```python
from build123d import *

# Parameters (mm, degrees)
F0_W     = 140
F0_H     = 15
F0_R     = 1.75
F1_DEPTH = 2.5
F3_DEPTH = 25
F4_W     = 18
F4_H     = 2.6
F4_W_2   = 12
F4_H_2   = 6
F4_W_3   = 10
F4_H_3   = 5
F5_DEPTH = 25
F6_D     = 3.4
F7_D     = 5.5
F8_R     = 5


with BuildPart() as f1:
    # F0 (on Top) → F1 (new body)
    with BuildSketch(Plane.XY):
        Rectangle(F0_W, F0_H)
        with Locations((-62, 0)):
            Circle(F0_R, mode=Mode.SUBTRACT)
        with Locations((62, 0)):
            Circle(F0_R, mode=Mode.SUBTRACT)
    extrude(amount=F1_DEPTH)

    # F2 (on face) → F3 (join)
    with BuildSketch(Plane.XY.offset(2.5)):
        Polygon((56.1840869486, 1.1), (-55.1196709275, 1.1), (-55.1196709275, -1.1), (56.1840869486, -1.1), (56.1840869486, 0), align=None)
    extrude(amount=F3_DEPTH)

    # F4 (on face) → F5 (cut)
    with BuildSketch(Plane(origin=(0, 1.1, 0), x_dir=(-1, 0, 0), z_dir=(0, 1, 0))):
        with Locations((42.6196709275, 16.3)):
            Rectangle(F4_W, F4_H)
        with Locations((42.6196709275, 13.7)):
            Rectangle(F4_W, F4_H)
        with Locations((15.6196709275, 18)):
            Rectangle(F4_W_2, F4_H_2)
        with Locations((15.6196709275, 12)):
            Rectangle(F4_W_2, F4_H_2)
        with Locations((-3.3803290725, 17.5)):
            Rectangle(F4_W_3, F4_H_3)
        with Locations((-3.3803290725, 12.5)):
            Rectangle(F4_W_3, F4_H_3)
    extrude(amount=-F5_DEPTH, mode=Mode.SUBTRACT)

    # F6 (through all)
    with Locations(Plane(origin=(0, 1.1, 0), x_dir=(-1, 0, 0), z_dir=(0, 1, 0))):
        with Locations((-51.1840869486, 15), (-46.1840869486, 15), (-16.1840869486, 9), (-26.1840869486, 9), (-36.1840869486, 9), (-51.1840869486, 9), (52.6196709275, 9), (40.6196709275, 9), (28.6196709275, 9)):
            Hole(F6_D / 2)

    # F7 (through all)
    with Locations(Plane(origin=(0, 1.1, 0), x_dir=(-1, 0, 0), z_dir=(0, 1, 0))):
        with Locations((-36.1840869486, 15), (-26.1840869486, 15), (-16.1840869486, 15), (-46.1840869486, 9), (47.6196709275, 9), (35.6196709275, 9)):
            Hole(F7_D / 2)

    # F8
    f8_edges = [f1.edges().sort_by_distance(p)[0] for p in [
        (56.184087, 0, 27.5),
        (-55.119671, 0, 27.5),
        (70, 7.5, 1.25),
        (70, -7.5, 1.25),
        (-70, 7.5, 1.25),
        (-70, -7.5, 1.25),
    ]]
    fillet(f8_edges, radius=F8_R)


solid = f1.part
```
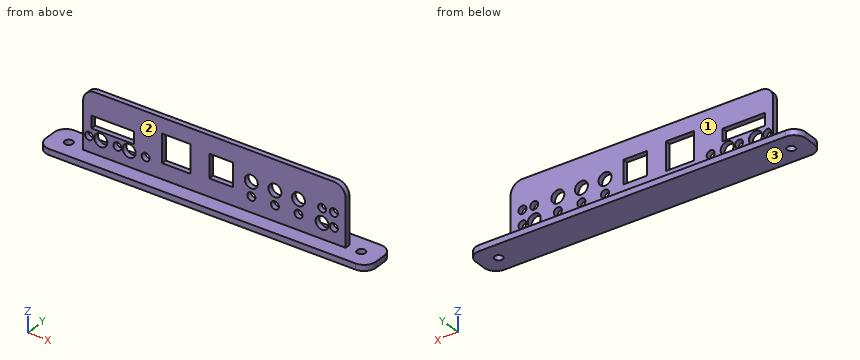
Geometry: final body of the model. Coordinates: model frame, mm. Face numbers are marked on the shaded views. Round coordinates to 2 decimals unless told otherwise and drop trailing zeros. Order: outer loops, then holes, each group sorted by start corner. A loop starts at its lowest first (then second) coordinate and runs counter-clockwise, first axis right, second up. Notation, with made-up numbers: (-38.5, -21.75) - (-15.5, -21.75) arc R23 ccw to (-15.5, 15.25) - close; hole circle Ø11 at (81, 40). An arc over 180 degrees is marked (long way). Use CSV: the item, a comma, the result in double quotes. Start each with the question number.
Q1. Section query B-B (y = -5.5). Return loops of the section in (x, z).
Q2. Mould query, pull axis Y, two halves, no side actions, for the marked faces 1, 2 and 3. Classes: +Y half, -Y half, draft (parallel to the pull), parting line (faces both ways), or undercut.
Q3. Section query D-D (x = 58.5). Return loops of the section in (y, z), and give its area (3 significant figures).
Q4. First-contact query: pin 1 (4 mm diameter, centred on x = -40.62, z = 9, fed in from -Y); pin 2 (2.5 mm diameter, centred on x = 51.18, z = 15, fed in from +Y); pin 3 (7.5 mm diameter, centred on x = -5.5, z = 13, fed in from +Y); pin 4 (5 mm diameter, centred on x = 35.5, y = -4, fed in from +Z). Flat tips, straight axial feed; report the tip coordinate or a pass-through.
Q5. Material intervals for line 1 along Z through (x, y) = (57, -1.75); line 2 along Y through (x, z) = (2, 9.5); line 3 along X through (y, z) = (6, 2), sorted ascending. Write a range as from..to.
Q6. Section query A-A (x = -62). Return loops of the section in (y, z), and give its area (4 significant figures).
Q7. Section query C-C (z = 15). State how many separate pieces and enclosed holes the cut face has, and give its area (3 significant figures).
Result set:
1,outline,"(-69, 0) - (69, 0) - (69, 2.5) - (-69, 2.5) - close"
2,face 1,"+Y half"
2,face 2,"-Y half"
2,face 3,"draft"
3,outline,"(-7.5, 0) - (7.5, 0) - (7.5, 2.5) - (-7.5, 2.5) - close"
3,area,"37.5 mm2"
4,pin 1,"stops at y = -1.1"
4,pin 2,"passes through"
4,pin 3,"stops at y = 1.1"
4,pin 4,"stops at z = 2.5"
5,line 1,"z = 0..2.5"
5,line 2,"y = -1.1..1.1"
5,line 3,"x = -68.57..68.57"
6,outline,"(-7.5, 0) - (-1.75, 0) - (-1.75, 2.5) - (-7.5, 2.5) - close; (1.75, 0) - (7.5, 0) - (7.5, 2.5) - (1.75, 2.5) - close"
6,area,"28.75 mm2"
7,separate pieces,"9"
7,enclosed holes,"0"
7,area,"106 mm2"
